Geometry check sheet. Reference: the model listing, model coordinates, mm. Face numbers are marked on the shaded views. Give positions to 0.01 mm unless a question says otherwise; leave off trailing zeros. Order: outer loops, then holes, each group sorted by start corner. A loop starts at its lowest first (then second) coordinate and runs counter-clockwise, first axis right, second up. Notation, with made-up numbers: M 3,23 L 9,23 A34 cw 9,57 Z; hole C -28.5,-29 d8. An arc over 180 degrees is marked long. One line per question, with ' | ' between items. Start each with the question number.
from build123d import *

# Parameters (mm, degrees)
SKETCH1_R           = 60.75
SKETCH1_R_2         = 45
BOSS_EXTRUDE1_DEPTH = 4
SKETCH2_R           = 49
SKETCH2_R_2         = 45
BOSS_EXTRUDE2_DEPTH = 52
SKETCH4_W           = 8
SKETCH4_H           = 41
SKETCH4_W_2         = 15
SKETCH4_H_2         = 8
BOSS_EXTRUDE3_DEPTH = 13
SKETCH6_W           = 10
SKETCH6_H           = 26
CUT_EXTRUDE1_DEPTH  = 26
SKETCH7_R           = 5
CUT_EXTRUDE2_DEPTH  = 110.592711893
SKETCH8_R           = 1.4
CUT_EXTRUDE7_DEPTH  = 7.2
BOSS_EXTRUDE4_DEPTH = 4
SKETCH12_R          = 2.5
CUT_EXTRUDE8_DEPTH  = 101.424723103


with BuildPart() as part:
    # Sketch1 → Boss-Extrude1 (new body)
    with BuildSketch(Plane(origin=(0, 0, 0), x_dir=(1, 0, 0), z_dir=(0, 1, 0))):
        with Locations(Location((0, 0, 0), (0, 0, 270))):
            Circle(SKETCH1_R)
        with Locations(Location((0, 0, 0), (0, 0, 270))):
            Circle(SKETCH1_R_2, mode=Mode.SUBTRACT)
    extrude(amount=BOSS_EXTRUDE1_DEPTH)

    # Sketch2 → Boss-Extrude2 (add)
    with BuildSketch(Plane(origin=(0, 4, 0), x_dir=(1, 0, 0), z_dir=(0, 1, 0))):
        with Locations(Location((0, 0, 0), (0, 0, 90))):
            Circle(SKETCH2_R)
        with Locations(Location((0, 0, 0), (0, 0, 270))):
            Circle(SKETCH2_R_2, mode=Mode.SUBTRACT)
    extrude(amount=BOSS_EXTRUDE2_DEPTH)

    # Sketch4 → Boss-Extrude3 (add, symmetric)
    with BuildSketch(Plane.XY):
        with Locations((15.25, 20.5)):
            Rectangle(SKETCH4_W, SKETCH4_H)
        with Locations((-39.25, 37)):
            Rectangle(SKETCH4_W_2, SKETCH4_H_2)
    extrude(amount=BOSS_EXTRUDE3_DEPTH, both=True)


with BuildPart() as boss_extrude3_piece_1:
    # of the separate pieces the step leaves, piece 1, a body of its own (boss_extrude3_pieces)
    add(part.part.solids().sort_by_distance((0, 0, 60.75))[0])

    # Sketch7 → Cut-Extrude2 (cut, through all)
    with BuildSketch(Plane.ZY.offset(-11.25)):
        with Locations(Location((0, 19, 0), (0, 0, 270))):
            Circle(SKETCH7_R)
    extrude(amount=-CUT_EXTRUDE2_DEPTH, mode=Mode.SUBTRACT)


with BuildPart() as boss_extrude3_piece_2:
    # of the separate pieces the step leaves, piece 2, a body of its own (boss_extrude3_pieces)
    add(part.part.solids().sort_by_distance((11.25, 41, -13))[0])

    # Sketch6 → Cut-Extrude1 (cut)
    with BuildSketch(Plane.ZY.offset(-11.25)):
        with Locations((0, 18)):
            Rectangle(SKETCH6_W, SKETCH6_H)
    extrude(amount=-CUT_EXTRUDE1_DEPTH, mode=Mode.SUBTRACT)


with BuildPart() as cut_extrude7_tool:
    # Sketch8 → Cut-Extrude7 (new body)
    with BuildSketch(Plane(origin=(0, 41, 0), x_dir=(1, 0, 0), z_dir=(0, 1, 0))):
        with Locations(Location((-34.25, -5, 0), (0, 0, 270))):
            Circle(SKETCH8_R)
        with Locations(Location((13.75, -5, 0), (0, 0, 270))):
            Circle(SKETCH8_R)
        with Locations(Location((13.75, 5, 0), (0, 0, 90))):
            Circle(SKETCH8_R)
        with Locations(Location((-34.25, 5, 0), (0, 0, 90))):
            Circle(SKETCH8_R)
    extrude(amount=-CUT_EXTRUDE7_DEPTH)


with BuildPart() as boss_extrude3_piece_1_1:
    add(boss_extrude3_piece_1.part)

    # Cut-Extrude7: cut by cut_extrude7_tool
    add(cut_extrude7_tool.part, mode=Mode.SUBTRACT)



with BuildPart() as boss_extrude3_piece_2_1:
    add(boss_extrude3_piece_2.part)

    # Cut-Extrude7: cut by cut_extrude7_tool
    add(cut_extrude7_tool.part, mode=Mode.SUBTRACT)


with BuildPart() as boss_extrude3_piece_1_2:
    add(boss_extrude3_piece_1_1.part)

    add(boss_extrude3_piece_2_1.part)  # Boss-Extrude4 merges Boss-Extrude3 piece 2
    # Sketch9 → Boss-Extrude4 (add)
    with BuildSketch(Plane.XZ):
        with BuildLine():
            Line((11.25, -13), (25.249838503, -37.248431585))
            ThreePointArc((25.249838503, -37.248431585), (45, 0), (25.249838503, 37.248431585))
            Line((25.249838503, 37.248431585), (11.25, 13))
            Line((11.25, 13), (19.25, 13))
            Line((19.25, 13), (19.25, -13))
            Line((19.25, -13), (11.25, -13))
        make_face()
        with BuildLine():
            ThreePointArc((27.361802413, -24.906460381), (37, 0), (27.361802413, 24.906460381))
            Line((27.361802413, 24.906460381), (24.25, 19.516660498))
            Line((24.25, 19.516660498), (24.25, -19.516660498))
            Line((24.25, -19.516660498), (27.361802413, -24.906460381))
        make_face(mode=Mode.SUBTRACT)
    extrude(amount=-BOSS_EXTRUDE4_DEPTH)

    # Sketch12 → Cut-Extrude8 (cut, through all)
    with BuildSketch(Plane(origin=(0, 4, 0), x_dir=(1, 0, 0), z_dir=(0, 1, 0))):
        with Locations(Location((-55, 0, 0), (0, 0, 270))):
            Circle(SKETCH12_R)
        with Locations(Location((0, 55, 0), (0, 0, 270))):
            Circle(SKETCH12_R)
        with Locations(Location((55, 0, 0), (0, 0, 270))):
            Circle(SKETCH12_R)
        with Locations(Location((0, -55, 0), (0, 0, 270))):
            Circle(SKETCH12_R)
    extrude(amount=-CUT_EXTRUDE8_DEPTH, mode=Mode.SUBTRACT)


solid = boss_extrude3_piece_1_2.part
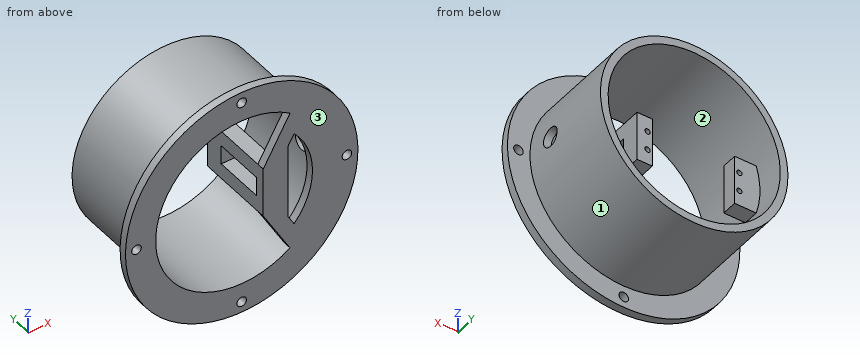
Item 1: Cross-section at B-B, the plane z = -55. Record the cut outline in (x, y).
Item 2: Depth check by flat-ended pin: pin 1 (1.5 mm diameter, centred on x = 40, z = -0.5, fed in from +Y); pin 2 (4 mm diameter, centred on x = 17, y = 12.5, fed in from -Z); pin 3 (4 mm diameter, centred on x = 45, y = 22.5, fed in from +Z). Enter the tip coordinate at first touch or a pass-through.
Item 3: Cross-section at D-D, the plane x = -41.5. Record the cut outline in (y, z).
Item 4: Cross-section at C-C, the plane y = 21. Record the cut outline in (x, z).
Item 5: Cross-section at A-A, the plane y = 39.5. Record the cut outline in (x, z).
Item 6: Material ranges on line 1 along Z through (x, y) = (-34, 35); line 2 along Z through (x, y) = (13, 37); line 3 along Y through (x, z) = (48, 0), recorded low to high.
Item 7: Mould release check, pull along Z, two halves, no side actions. Record for the marked faces 1, 2 and 3: released by +Z, released by -Z, zero draft, split by the parting line, or undercut.
Outcome:
1) outline: M -25.8,0 L -2.5,0 L -2.5,4 L -25.8,4 Z; M 2.5,0 L 25.8,0 L 25.8,4 L 2.5,4 Z
2) pin 1: stops at y = 4 | pin 2: stops at z = -46.65 | pin 3: stops at z = 23.49
3) outline: M 0,-44.37 L 4,-44.37 L 4,-26.05 L 56,-26.05 L 56,-17.4 L 0,-17.4 Z; M 0,17.4 L 56,17.4 L 56,26.05 L 4,26.05 L 4,44.37 L 0,44.37 Z; M 33,-13 L 41,-13 L 41,13 L 33,13 Z
4) outline: M 11.25,-13 L 19.25,-13 L 19.25,-5 L 11.25,-5 Z; M 11.25,5 L 19.25,5 L 19.25,13 L 11.25,13 Z; M 44.77,-4.58 A45 cw long 44.77,4.58 L 48.79,4.58 A49 ccw long 48.79,-4.58 Z
5) outline: C 0,0 d98; M 11.25,-13 L 19.25,-13 L 19.25,13 L 11.25,13 Z; hole M -43.08,-13 A45 ccw long -43.08,13 L -31.75,13 L -31.75,-13 Z; hole C -34.25,-5 d2.8; hole C -34.25,5 d2.8; hole C 13.75,-5 d2.8; hole C 13.75,5 d2.8
6) line 1: z = -35.28 to -29.48, -13 to -6.38, -3.62 to 3.62, 6.38 to 13, 29.48 to 35.28 | line 2: z = -47.24 to -43.08, -13 to -6.18, -3.82 to 3.82, 6.18 to 13, 43.08 to 47.24 | line 3: y = 0 to 14, 24 to 56
7) face 1: split by the parting line | face 2: undercut | face 3: zero draft
